```python
from build123d import *

# Parameters (mm, degrees)
SKETCH_1_R          = 3
SKETCH_1_W          = 40
SKETCH_1_H          = 20
EXTRUDE_1_DEPTH     = 4
EXTRUDE_3_DEPTH     = 4
SKETCH_3_R          = 3
EXTRUDE_4_DEPTH     = 4
SKETCH_4_R          = 1
CUT_EXTRUDE_1_DEPTH = 4
SKETCH_5_R          = 1
CUT_EXTRUDE_2_DEPTH = 5
SKETCH_6_W          = 5
SKETCH_6_H          = 7
SKETCH_6_W_2        = 40.5
SKETCH_6_H_2        = 20
SKETCH_6_R          = 1
SKETCH_6_W_3        = 22
SKETCH_6_H_3        = 12
CUT_EXTRUDE_3_DEPTH = 10


with BuildPart() as part:
    # 草图1 → 凸台-拉伸1 (new body)
    with BuildSketch(Plane.XY):
        with BuildLine():
            ThreePointArc((-45, -15), (-42.071067812, -22.071067812), (-35, -25))
            Line((-35, -25), (35, -25))
            ThreePointArc((35, -25), (42.071067812, -22.071067812), (45, -15))
            Line((45, -15), (45, -6.75))
            Line((45, -6.75), (30, -6.75))
            ThreePointArc((30, -6.75), (28.25, -5), (30, -3.25))
            Line((30, -3.25), (45, -3.25))
            Line((45, -3.25), (45, 8.25))
            Line((45, 8.25), (35, 8.25))
            ThreePointArc((35, 8.25), (33.25, 10), (35, 11.75))
            Line((35, 11.75), (45, 11.75))
            Line((45, 11.75), (45, 15))
            ThreePointArc((45, 15), (42.071067812, 22.071067812), (35, 25))
            Line((35, 25), (-35, 25))
            ThreePointArc((-35, 25), (-42.071067812, 22.071067812), (-45, 15))
            Line((-45, 15), (-45, 11.75))
            Line((-45, 11.75), (-35, 11.75))
            ThreePointArc((-35, 11.75), (-33.25, 10), (-35, 8.25))
            Line((-35, 8.25), (-45, 8.25))
            Line((-45, 8.25), (-45, -3.25))
            Line((-45, -3.25), (-30, -3.25))
            ThreePointArc((-30, -3.25), (-28.25, -5), (-30, -6.75))
            Line((-30, -6.75), (-45, -6.75))
            Line((-45, -6.75), (-45, -15))
        make_face()
        with BuildLine():
            ThreePointArc((-20, -18), (-23, -15), (-20, -12))
            Line((-20, -12), (20, -12))
            ThreePointArc((20, -12), (23, -15), (20, -18))
            Line((20, -18), (-20, -18))
        make_face(mode=Mode.SUBTRACT)
        with Locations((-24, 0)):
            Circle(SKETCH_1_R, mode=Mode.SUBTRACT)
        with Locations((-24, 10)):
            Circle(SKETCH_1_R, mode=Mode.SUBTRACT)
        with Locations((0, 5)):
            Rectangle(SKETCH_1_W, SKETCH_1_H, mode=Mode.SUBTRACT)
        with Locations((24, 0)):
            Circle(SKETCH_1_R, mode=Mode.SUBTRACT)
        with Locations((24, 10)):
            Circle(SKETCH_1_R, mode=Mode.SUBTRACT)
    extrude(amount=EXTRUDE_1_DEPTH)

    # 草图2 → 凸台-拉伸3 (add)
    with BuildSketch(Plane.XY.offset(4)):
        Polygon((20, -5), (20, 5), (11, 5), (11, -1), (-11, -1), (-11, 5), (-20, 5), (-20, -5), align=None)
        Polygon((11, 5), (20, 5), (20, 15), (-20, 15), (-20, 5), (-11, 5), (-11, 11), (11, 11), align=None)
    extrude(amount=-EXTRUDE_3_DEPTH)

    # 草图3 → 凸台-拉伸4 (add)
    with BuildSketch(Plane.XY.offset(4)):
        with Locations((-24, 10)):
            Circle(SKETCH_3_R)
        with Locations((-24, 0)):
            Circle(SKETCH_3_R)
        with Locations((24, 10)):
            Circle(SKETCH_3_R)
        with Locations((24, 0)):
            Circle(SKETCH_3_R)
    extrude(amount=-EXTRUDE_4_DEPTH)

    # 草图4 → 切除-拉伸1 (cut)
    with BuildSketch(Plane.XY.offset(4)):
        with Locations((-14, 5)):
            Circle(SKETCH_4_R)
        with Locations((14, 5)):
            Circle(SKETCH_4_R)
    extrude(amount=-CUT_EXTRUDE_1_DEPTH, mode=Mode.SUBTRACT)

    # 草图5 → 切除-拉伸2 (cut, through all)
    with BuildSketch(Plane.XY.offset(4)):
        with Locations((-22.5, -3)):
            Circle(SKETCH_5_R)
        with Locations((-22.5, 13)):
            Circle(SKETCH_5_R)
    cut_extrude_2 = extrude(amount=-CUT_EXTRUDE_2_DEPTH, mode=Mode.SUBTRACT)

    # 镜向1: 切除-拉伸2 across plane
    add(cut_extrude_2.mirror(Plane(origin=(0, 0, 0), x_dir=(0, 0, 1), z_dir=(1, 0, 0))), mode=Mode.SUBTRACT)

    # 草图6 → 切除-拉伸3 (cut)
    with BuildSketch(Plane.XY.offset(4)):
        with Locations((-22.75, 5)):
            Rectangle(SKETCH_6_W, SKETCH_6_H)
        with Locations((0, 5)):
            Rectangle(SKETCH_6_W_2, SKETCH_6_H_2)
        with Locations((14, 5)):
            Circle(SKETCH_6_R, mode=Mode.SUBTRACT)
        with Locations((-14, 5)):
            Circle(SKETCH_6_R, mode=Mode.SUBTRACT)
        with Locations((0, 5)):
            Rectangle(SKETCH_6_W_3, SKETCH_6_H_3, mode=Mode.SUBTRACT)
    extrude(amount=-CUT_EXTRUDE_3_DEPTH, mode=Mode.SUBTRACT)


solid = part.part
```
Geometry: final body of the model. Coordinates: model frame, mm. A direction names the side the tool comes from. Round coordinates to 2 decimals unless told otherwise and drop trailing zeros. Loops run counter-clockwise (first coordinate to the right, second up) from the corner with the lowest first, then second, coordinate; pieces in that order, holes last.
Item 1: Section B-B, the plane x = 2.5. Output: boundary loops of the cut face in (y, z).
Checked values:
outline: (-25, 0) - (-18, 0) - (-18, 4) - (-25, 4) - close; (-12, 0) - (-5, 0) - (-5, 4) - (-12, 4) - close; (15, 0) - (25, 0) - (25, 4) - (15, 4) - close
Item 2: Section A-A, the plane y = 5. Output: boundary loops of the cut face in (x, z).
Checked values:
outline: (-45, 0) - (-25.25, 0) - (-25.25, 4) - (-45, 4) - close; (20.25, 0) - (45, 0) - (45, 4) - (20.25, 4) - close
Item 3: Line query: L1, parallel to Y at x = 17, z = 0.4; L2, parallel to X at y = 6, z = 2.7; L3, parallel to Y at x = 37, z = 1.7. Output: solid intervals per line, ascending.
Checked values:
L1: y = -25 to -18, -12 to -5, 15 to 25
L2: x = -45 to -25.25, 20.25 to 45
L3: y = -24.8 to -6.75, -3.25 to 8.25, 11.75 to 24.8
Item 4: Contact query for flat-ended pins moving along their axis: P1, Ø2, axis at x = -37.5, z = 1.5, coming from the -Y side; P2, Ø2, axis at y = 11.5, z = 2.5, coming from the +X side; P3, Ø1.6, axis at x = -22.5, y = 13, coming from the -Z side; P4, Ø2, axis at x = 38.5, z = 3, coming from the -Y side. Output: stop coordinate, or through.
Checked values:
P1: stops at y = -24.89
P2: stops at x = 45
P3: passes through
P4: stops at y = -24.68
Item 5: Section C-C, the plane y = 10. Output: boundary loops of the cut face in (x, z), plus the area to 3 significant figures.
Checked values:
outline: (-33.25, 0) - (-20.25, 0) - (-20.25, 4) - (-33.25, 4) - close; (20.25, 0) - (33.25, 0) - (33.25, 4) - (20.25, 4) - close
area: 104 mm2
Item 6: Section D-D, the plane z = 1.45. State how many separate pieces and enclosed holes the cut face has, plus the area to 3 significant figures.
Checked values:
separate pieces: 1
enclosed holes: 6
area: 3,090 mm2
Item 7: Reachability of faces 1 (the flat face through (-25.25, 5, 2)), 2 (the flat face through (37, -3.25, 2)), 3 (the flat face through (45, 2, 2)) from +Z, -Z, +X, -X, +Y, -Y: full face, straight path, thin tool, end or side. Return the list, or none.
Checked values:
face 1: +Z, -Z
face 2: +Z, -Z, +X
face 3: +Z, -Z, +X, +Y, -Y
